```python
from build123d import *

# Parameters (mm, degrees)
F0_W     = 189
F0_H     = 119
F1_DEPTH = 268
F2_T     = -3
F4_DEPTH = 268
F6_DEPTH = 189


with BuildPart() as f1:
    # F0 (on Front) → F1 (new body)
    with BuildSketch(Plane.XZ):
        with Locations((94.5, 59.5)):
            Rectangle(F0_W, F0_H)
    extrude(amount=F1_DEPTH)

    # F2
    f2_openings = [f1.faces().sort_by_distance(p)[0] for p in [
        (94.5, -134, 119),
    ]]
    offset(amount=F2_T, openings=f2_openings)

    # F3 (on face) → F4 (join, through all)
    with BuildSketch(Plane.XZ.offset(268)):
        with BuildLine():
            Line((-77.942286, 74), (0, 119))
            Line((0, 119), (3.464102, 119))
            ThreePointArc((3.464102, 119), (2.44949, 121.44949), (0, 122.464102))
            Line((0, 122.464102), (-79.442286, 76.598076))
            Line((-79.442286, 76.598076), (-77.942286, 74))
        make_face()
        with BuildLine():
            Line((185.535898, 119), (189, 119))
            Line((189, 119), (266.942286, 164))
            Line((266.942286, 164), (265.442286, 166.598076))
            Line((265.442286, 166.598076), (189, 122.464102))
            ThreePointArc((189, 122.464102), (186.55051, 121.44949), (185.535898, 119))
        make_face()
    extrude(amount=-F4_DEPTH)

    # F5 (on face) → F6 (join, through all)
    with BuildSketch(Plane(origin=(0, 0, 0), x_dir=(0, -1, 0), z_dir=(-1, 0, 0))):
        with BuildLine():
            Line((264.535898, 119), (268, 119))
            Line((268, 119), (345.942286, 74))
            Line((345.942286, 74), (347.442286, 76.598076))
            Line((347.442286, 76.598076), (268, 122.464102))
            ThreePointArc((268, 122.464102), (265.55051, 121.44949), (264.535898, 119))
        make_face()
        with BuildLine():
            Line((-77.942286, 164), (0, 119))
            Line((0, 119), (3.464102, 119))
            ThreePointArc((3.464102, 119), (2.44949, 121.44949), (0, 122.464102))
            Line((0, 122.464102), (-76.442286, 166.598076))
            Line((-76.442286, 166.598076), (-77.942286, 164))
        make_face()
    extrude(amount=-F6_DEPTH)


solid = f1.part
```
Verification items for the finished model (mm, model axes). A direction names the side the tool comes from. Give positions to 0.01 mm unless a question says otherwise; leave off trailing zeros. Order: outer loops, then holes, each group sorted by start corner. A loop starts at its lowest first (then second) coordinate and runs counter-clockwise, first axis right, second up. Notation, with made-up numbers: M -19,8.5 L 7,8.5 A31 ccw 7,36.5 Z; hole C 67.25,80.5 d6. An arc over 180 degrees is marked long. Answer in a Markdown table with one row per item. Add a question column.
Item 1: Gauge pin test, flat ends, axial feed: pin 1 (5 mm diameter, centred on x = 71, z = 17, fed in from +Y); pin 2 (6 mm diameter, centred on x = 20.5, y = -263, fed in from +Z); pin 3 (1 mm diameter, centred on y = -33, z = 65, fed in from +X). Record the tip position at first contact, or that the pin passes through.
Item 2: Mould release check, pull along Y, two halves, no side actions. Record for faces 5 (the flat face through (93.177, 37.686, 144.222)), 6 (the flat face through (189, -132, 59)), 7 (the flat face through (93, -3, 62)), 8 (the flat face through (93.177, -306.426, 96.815)): released by +Y, released by -Y, zero draft, split by the parting line, or undercut.
Item 3: Scan lines: probe 1 along X at (y, z) = (-211.5, 64); probe 2 along Y at (x, z) = (74, 34); probe 3 along Y at (x, z) = (48.5, 102). Record each from-to range of solid material in increasing order. Write a range as from..to.
Item 4: Section check A-A, the plane z = 18.5. Enter the section's corners in (x, y).
Item 5: Tool access check on faces 1 (the flat face through (3, -132, 60)), 2 (the flat face through (93, -268, 60)), 3 (the flat face through (0, -132, 59)), 4 (the flat face through (93, 0, 60)). Record the directions out of +Z, -Z, +X, -X, +Y, -Y that give a thin tool (end or side, any length) a straight path to the whole face; none if there is none.
Item 6: Section check D-D, the plane x = 99. Enter the section's corners in (y, z).
Item 7: Section check B-B, the plane y = -217. Enter the section's corners in (x, z).
Item 8: Section check C-C, the plane z = 109. Enter the section's corners in (x, y).
Filled sheet:
| question | item | result |
|---|---|---|
| 1 | pin 1 | stops at y = 0 |
| 1 | pin 2 | stops at z = 121.83 |
| 1 | pin 3 | stops at x = 189 |
| 2 | face 5 | released by -Y |
| 2 | face 6 | zero draft |
| 2 | face 7 | undercut |
| 2 | face 8 | undercut |
| 3 | probe 1 | x = 0..3, 186..189 |
| 3 | probe 2 | y = -268..-265, -3..0 |
| 3 | probe 3 | y = -303.44..-297.44, -268..-265, -3..0 |
| 4 | outline | M 0,-268 L 189,-268 L 189,0 L 0,0 Z; hole M 3,-265 L 186,-265 L 186,-3 L 3,-3 Z |
| 5 | face 1 | none |
| 5 | face 2 | -Z, +X, -X |
| 5 | face 3 | -Z, +Y, -Y |
| 5 | face 4 | -Z, +X, -X, +Y |
| 6 | outline | M -347.44,76.6 L -345.94,74 L -268,119 L -268,0 L 0,0 L 0,119 L 77.94,164 L 76.44,166.6 L 0,122.46 A3.46 ccw -3.46,119 L -3,119 L -3,3 L -265,3 L -265,119 L -264.54,119 A3.46 ccw -268,122.46 Z |
| 7 | outline | M -79.44,76.6 L -77.94,74 L 0,119 L 0,0 L 189,0 L 189,119 L 266.94,164 L 265.44,166.6 L 189,122.46 A3.46 ccw 185.54,119 L 186,119 L 186,3 L 3,3 L 3,119 L 3.46,119 A3.46 ccw 0,122.46 Z |
| 8 | outline | M -23.32,-268 L -17.32,-268 L -17.32,0 L -23.32,0 Z; M 0,-291.32 L 189,-291.32 L 189,-285.32 L 0,-285.32 Z; M 0,-268 L 189,-268 L 189,0 L 0,0 Z; hole M 3,-265 L 186,-265 L 186,-3 L 3,-3 Z |
